The listing builds one solid part. Answer for the finished solid, in the listing's coordinates (mm). A direction names the side the tool comes from. Give positions to 0.01 mm unless a question says otherwise; leave off trailing zeros. Order: outer loops, then holes, each group sorted by start corner. A loop starts at its lowest first (then second) coordinate and runs counter-clockwise, first axis right, second up. Notation, with made-up numbers: M 25.5,65 L 46.5,65 A25 cw 46.5,93 Z; hole C -24,37.5 d7. An arc over 180 degrees is marked long. Answer as a JSON object with one key per item and string values. Group by question number.
```python
from build123d import *

# Parameters (mm, degrees)
ESBO_O1_R                          = 6
ESBO_O1_R_2                        = 1.25
RESSALTO_EXTRUS_O1_DEPTH           = 5
ESBO_O2_W                          = 5.8
ESBO_O2_H                          = 12.09
RESSALTO_EXTRUS_O2_DEPTH           = 22
REBAIXO_PARA_SBHCS_M31_D           = 3.2
REBAIXO_PARA_SBHCS_M31_DEPTH       = 5.8
REBAIXO_PARA_SBHCS_M31_CBORE_D     = 6.7
REBAIXO_PARA_SBHCS_M31_CBORE_DEPTH = 1.65
FILETE1_R                          = 5


with BuildPart() as part:
    # Esboço1 → Ressalto-extrusão1 (new body)
    with BuildSketch(Plane.XY):
        with BuildLine():
            Line((-14.25, 2.165063509), (5.25, 13.423393759))
            ThreePointArc((5.25, 13.423393759), (7.75, 13.423393759), (9, 11.258330249))
            Line((9, 11.258330249), (9, -11.258330249))
            Line((9, -11.258330249), (9, -31.498330249))
            Line((9, -31.498330249), (3.2, -31.498330249))
            Line((3.2, -31.498330249), (3.2, -19.408330249))
            Line((3.2, -19.408330249), (3.2, -18.013328399))
            ThreePointArc((3.2, -18.013328399), (1.860254038, -13.013328399), (-1.8, -9.353074361))
            Line((-1.8, -9.353074361), (-14.25, -2.165063509))
            ThreePointArc((-14.25, -2.165063509), (-15.5, 0), (-14.25, 2.165063509))
        make_face()
        Circle(ESBO_O1_R, mode=Mode.SUBTRACT)
        with Locations((6.5, -11.258330249)):
            Circle(ESBO_O1_R_2, mode=Mode.SUBTRACT)
        with Locations((6.5, 11.258330249)):
            Circle(ESBO_O1_R_2, mode=Mode.SUBTRACT)
        with Locations((-13, 0)):
            Circle(ESBO_O1_R_2, mode=Mode.SUBTRACT)
    extrude(amount=RESSALTO_EXTRUS_O1_DEPTH)

    # Esboço2 → Ressalto-extrusão2 (add)
    with BuildSketch(Plane(origin=(0, 0, 0), x_dir=(-1, 0, 0), z_dir=(0, 0, -1))):
        with Locations((-6.1, -25.453330249)):
            Rectangle(ESBO_O2_W, ESBO_O2_H)
    extrude(amount=RESSALTO_EXTRUS_O2_DEPTH)

    # Rebaixo para SBHCS M31
    with Locations(Plane(origin=(9, 0, 0), x_dir=(0, 0, -1), z_dir=(1, 0, 0))):
        with Locations((1, -25.453330249), (16, -25.453330249)):
            CounterBoreHole(REBAIXO_PARA_SBHCS_M31_D / 2, REBAIXO_PARA_SBHCS_M31_CBORE_D / 2, REBAIXO_PARA_SBHCS_M31_CBORE_DEPTH, depth=REBAIXO_PARA_SBHCS_M31_DEPTH)

    # Filete1
    filete1_edges = [part.edges().sort_by_distance(p)[0] for p in [
        (6.1, -19.408330249, 0),
    ]]
    fillet(filete1_edges, radius=FILETE1_R)


solid = part.part
```
Item 1: A tool of negligible diameter and unlimited length cuts with its end or side. For faces 4 (the cylindrical face through (-6, 0, 2)), 5 (the flat face through (-0.4, -6.4, 0)), 6 (the cylindrical face through (8.187, -28.724, -15.274)), 7 (the flat face through (3.2, -25, -8)), from which of +Z, -Z, +X, -X, +Y, -Y can it reach the whole face along a straight path? Write none if from no direction.
Item 2: Section A-A (x = 6.5) is taken. Determine the outline of the cut face in (y, z).
Item 3: Section B-B (y = 0) is taken. Determine the outline of the cut face in (x, z), and give its area (3 significant figures).
Item 4: Consider probe 1 along Y at (x, z) = (6.5, 2.75); probe 2 along Y at (x, z) = (8.25, -16); probe 3 along X at (y, z) = (-27.5, 1.5). Determine where each line is inside the solid, lowest interval first. Write a range as from..to.
Item 5: Section D-D (x = -12.25) is taken. Determine the outline of the cut face in (y, z), and give its area (3 significant figures).
Item 6: Section C-C (z = -16) is taken. Determine the outline of the cut face in (x, y).
Item 7: Flat-ended cylindrical pins translate along their axes: P1, Ø6, axis at y = -25.45, z = -16, coming from the -X side; P2, Ø7.5, axis at x = 0.5, y = -4, coming from the -Z side; P3, Ø2, axis at y = -25, z = 0, coming from the +X side. Find the tip coordinate at first contact, or state that the pin passes through.
Item 8: Determine the mould class of faces 1 (the cylindrical face through (-14.25, 0.05, 2.46)), 2 (the flat face through (9, -20, -5)), 3 (the cylindrical face through (-15.5, 0, 2.5)) for opening direction Y: released by +Y, released by -Y, zero draft, split by the parting line, or undercut.
Values found:
{
 "1": {"face 4": "+Z, -Z", "face 5": "-Z, +X, -X, +Y", "face 6": "+X", "face 7": "+Z, -Z, -X, -Y"},
 "2": {"outline": "M -31.5,-22 L -19.41,-22 L -19.41,-5 A5 cw -14.41,0 L -12.51,0 L -12.51,5 L -31.5,5 Z; M -10.01,0 L 10.01,0 L 10.01,5 L -10.01,5 Z; M 12.51,0 L 13.76,0 L 13.76,5 L 12.51,5 Z; hole C -25.45,-16 d3.2; hole C -25.45,-1 d3.2"},
 "3": {"outline": "M -15.5,0 L -14.25,0 L -14.25,5 L -15.5,5 Z; M -11.75,0 L -6,0 L -6,5 L -11.75,5 Z; M 6,0 L 9,0 L 9,5 L 6,5 Z", "area": "50.0 mm^2"},
 "4": {"probe 1": "y = -31.5..-12.51, -10.01..10.01, 12.51..13.76", "probe 2": "y = -31.5..-28.8, -22.1..-19.41", "probe 3": "x = 3.2..7.35"},
 "5": {"outline": "M -3.32,0 L -1,0 L -1,5 L -3.32,5 Z; M 1,0 L 3.32,0 L 3.32,5 L 1,5 Z", "area": "23.2 mm^2"},
 "6": {"outline": "M 3.2,-31.5 L 9,-31.5 L 9,-28.8 L 7.35,-28.8 L 7.35,-27.05 L 3.2,-27.05 Z; M 3.2,-23.85 L 7.35,-23.85 L 7.35,-22.1 L 9,-22.1 L 9,-19.41 L 3.2,-19.41 Z"},
 "7": {"P1": "stops at x = 3.2", "P2": "stops at z = 0", "P3": "stops at x = 7.35"},
 "8": {"face 1": "undercut", "face 2": "zero draft", "face 3": "split by the parting line"}
}
